Input: part model. Units: mm. Frame: model coordinates. A direction names the side the tool comes from. Round coordinates to 2 decimals unless told otherwise and drop trailing zeros. Order: outer loops, then holes, each group sorted by start corner. A loop starts at its lowest first (then second) coordinate and runs counter-clockwise, first axis right, second up. Notation, with made-up numbers: (70, 79) -> (113, 79) arc R33 ccw to (113, 108) -> close; hole circle Ø2 at (-18.5, -32). An arc over 180 degrees is marked (long way). Use a Markdown table: item, result.
from build123d import *

# Parameters (mm, degrees)
SKETCH_1_R            = 21.5
SKETCH_1_R_2          = 1.5
SKETCH_1_R_3          = 10
EXTRUDE_1_DEPTH       = 9
SHELL_4_T             = -2
EXTRUDE_2_OUTLINE_R   = 21.5
EXTRUDE_2_OUTLINE_R_2 = 1.5
EXTRUDE_2_OUTLINE_R_3 = 4
EXTRUDE_2_DEPTH       = 3
SKETCH_5_R            = 13.5
SKETCH_5_R_2          = 1.5
SKETCH_5_R_3          = 4
EXTRUDE_3_DEPTH       = 3


# Read off the part's stored shape, not the designer's step: 凸台-拉伸2
with BuildPart() as part:
    # 草图1 → 凸台-拉伸1 (new body)
    with BuildSketch(Plane(origin=(0, 0, 0), x_dir=(1, 0, 0), z_dir=(0, 1, 0))):
        with Locations(Location((0, 0, 0), (0, 0, 270))):
            Circle(SKETCH_1_R)
        with Locations(Location((12.374368671, 12.374368671, 0), (0, 0, 270))):
            Circle(SKETCH_1_R_2, mode=Mode.SUBTRACT)
        with Locations(Location((0, 0, 0), (0, 0, 270))):
            Circle(SKETCH_1_R_3, mode=Mode.SUBTRACT)
        with Locations(Location((12.374368671, -12.374368671, 0), (0, 0, 90))):
            Circle(SKETCH_1_R_2, mode=Mode.SUBTRACT)
        with Locations(Location((-12.374368671, -12.374368671, 0), (0, 0, 270))):
            Circle(SKETCH_1_R_2, mode=Mode.SUBTRACT)
        with Locations(Location((-12.374368671, 12.374368671, 0), (0, 0, 90))):
            Circle(SKETCH_1_R_2, mode=Mode.SUBTRACT)
        with Locations(Location((0, 17.5, 0), (0, 0, 90))):
            Circle(SKETCH_1_R_2, mode=Mode.SUBTRACT)
        with Locations(Location((17.5, 0, 0), (0, 0, 270))):
            Circle(SKETCH_1_R_2, mode=Mode.SUBTRACT)
        with Locations(Location((0, -17.5, 0), (0, 0, 90))):
            Circle(SKETCH_1_R_2, mode=Mode.SUBTRACT)
        with Locations(Location((-17.5, 0, 0), (0, 0, 270))):
            Circle(SKETCH_1_R_2, mode=Mode.SUBTRACT)
    extrude(amount=EXTRUDE_1_DEPTH)

    # 抽壳4
    shell_4_openings = [part.faces().sort_by_distance(p)[0] for p in [
        (0, 9, -20.891888168),
    ]]
    offset(amount=SHELL_4_T, openings=shell_4_openings, kind=Kind.INTERSECTION)

    # 凸台-拉伸2 outline → 凸台-拉伸2 (add)
    with BuildSketch(Plane(origin=(0, 9, 0), x_dir=(1, 0, 0), z_dir=(0, 1, 0))):
        Circle(EXTRUDE_2_OUTLINE_R)
        with Locations((-12.374368671, -12.374368671)):
            Circle(EXTRUDE_2_OUTLINE_R_2, mode=Mode.SUBTRACT)
        with Locations((0, -17.5)):
            Circle(EXTRUDE_2_OUTLINE_R_2, mode=Mode.SUBTRACT)
        with Locations((12.374368671, -12.374368671)):
            Circle(EXTRUDE_2_OUTLINE_R_2, mode=Mode.SUBTRACT)
        with Locations((0, -7)):
            Circle(EXTRUDE_2_OUTLINE_R_2, mode=Mode.SUBTRACT)
        with Locations((-17.5, 0)):
            Circle(EXTRUDE_2_OUTLINE_R_2, mode=Mode.SUBTRACT)
        with Locations((-7, 0)):
            Circle(EXTRUDE_2_OUTLINE_R_2, mode=Mode.SUBTRACT)
        with Locations((-12.374368671, 12.374368671)):
            Circle(EXTRUDE_2_OUTLINE_R_2, mode=Mode.SUBTRACT)
        Circle(EXTRUDE_2_OUTLINE_R_3, mode=Mode.SUBTRACT)
        with Locations((7, 0)):
            Circle(EXTRUDE_2_OUTLINE_R_2, mode=Mode.SUBTRACT)
        with Locations((0, 7)):
            Circle(EXTRUDE_2_OUTLINE_R_2, mode=Mode.SUBTRACT)
        with Locations((17.5, 0)):
            Circle(EXTRUDE_2_OUTLINE_R_2, mode=Mode.SUBTRACT)
        with Locations((0, 17.5)):
            Circle(EXTRUDE_2_OUTLINE_R_2, mode=Mode.SUBTRACT)
        with Locations((12.374368671, 12.374368671)):
            Circle(EXTRUDE_2_OUTLINE_R_2, mode=Mode.SUBTRACT)
    extrude(amount=EXTRUDE_2_DEPTH)

    # 草图5 → 凸台-拉伸3 (add)
    with BuildSketch(Plane(origin=(0, 12, 0), x_dir=(1, 0, 0), z_dir=(0, 1, 0))):
        with Locations(Location((0, 0, 0), (0, 0, 270))):
            Circle(SKETCH_5_R)
        with Locations(Location((-7, 0, 0), (0, 0, 270))):
            Circle(SKETCH_5_R_2, mode=Mode.SUBTRACT)
        with Locations(Location((0, -7, 0), (0, 0, 270))):
            Circle(SKETCH_5_R_2, mode=Mode.SUBTRACT)
        with Locations(Location((7, 0, 0), (0, 0, 270))):
            Circle(SKETCH_5_R_2, mode=Mode.SUBTRACT)
        with Locations(Location((0, 0, 0), (0, 0, 270))):
            Circle(SKETCH_5_R_3, mode=Mode.SUBTRACT)
        with Locations(Location((0, 7, 0), (0, 0, 270))):
            Circle(SKETCH_5_R_2, mode=Mode.SUBTRACT)
    extrude(amount=EXTRUDE_3_DEPTH)


solid = part.part
1) Set-up query: faces 5 (the face through (0.56, 12.62, 8.39)), 6 (the face through (18.04, 5.45, -7.4)), 7 (the face through (3, 15, 3)), 8 (the face through (-13.18, 13.48, -2.93)), 9 (the face through (-0.1, 9, 4.3)). Return all of +Z, -Z, +X, -X, +Y, -Y with unobstructed straight access to the full face (end or side cutting, diameter ignored); none if empty.
Answer key:
| item | result |
|---|---|
| face 5 | +Y, -Y |
| face 6 | none |
| face 7 | +Z, -Z, +X, -X, +Y |
| face 8 | +Y |
| face 9 | -Y |
2) Ray query, probe 1 along X at (y, z) = (13.65, 0); probe 2 along X at (y, z) = (10.35, 0); probe 3 along Y at (x, z) = (2, 13). Return the intervals inside material, ascending.
Answer key:
| item | result |
|---|---|
| probe 1 | x = -13.5 to -8.5, -5.5 to -4, 4 to 5.5, 8.5 to 13.5 |
| probe 2 | x = -21.5 to -19, -16 to -8.5, -5.5 to -4, 4 to 5.5, 8.5 to 16, 19 to 21.5 |
| probe 3 | y = 0 to 2, 9 to 15 |
3) Cut plane C-C on y = 10. State how many separate pieces and enclosed holes the cut face has, and give its area (3 significant figures).
Answer key:
| item | result |
|---|---|
| separate pieces | 1 |
| enclosed holes | 13 |
| area | 1,320 mm^2 |
4) Cut plane B-B on z = -17.5. Return loops of the section in (x, y), and give its area (3 significant figures).
Answer key:
| item | result |
|---|---|
| outline | (-12.49, 0) -> (-1.5, 0) -> (-1.5, 12) -> (-12.49, 12) -> close; (1.5, 0) -> (12.49, 0) -> (12.49, 12) -> (1.5, 12) -> close; hole (-8.6, 2) -> (-3.5, 2) -> (-3.5, 9) -> (-8.6, 9) -> close; hole (3.5, 2) -> (8.6, 2) -> (8.6, 9) -> (3.5, 9) -> close |
| area | 192 mm^2 |
5) Draft query along Y for faces 1 (the face through (-18.04, 5.45, 7.4)), 2 (the face through (-9.76, 4.44, -2.17)), 3 (the face through (-4.5, 0, 9.3)), 4 (the face through (18, 5.5, 7.5)). Return one class per face: released by +Y, released by -Y, zero draft, split by the parting line, or undercut.
Answer key:
| item | result |
|---|---|
| face 1 | undercut |
| face 2 | zero draft |
| face 3 | released by -Y |
| face 4 | undercut |
6) Cut plane A-A on x = -7. Return loops of the section in (y, z).
Answer key:
| item | result |
|---|---|
| outline | (0, -20.33) -> (12, -20.33) -> (12, -11.54) -> (15, -11.54) -> (15, -1.5) -> (9, -1.5) -> (9, -7.14) -> (0, -7.14) -> close; (0, 7.14) -> (9, 7.14) -> (9, 1.5) -> (15, 1.5) -> (15, 11.54) -> (12, 11.54) -> (12, 20.33) -> (0, 20.33) -> close; hole (2, -18.2) -> (9, -18.2) -> (9, -9.75) -> (2, -9.75) -> close; hole (2, 9.75) -> (9, 9.75) -> (9, 18.2) -> (2, 18.2) -> close |
7) Contact query for flat-ended pins moving along their axis: P1, Ø16, axis at x = 3, z = 1.5, coming from the -Y side; P2, Ø3, axis at x = 6, y = 11, coming from the +Z side; P3, Ø4, axis at x = -5, z = -16, coming from the +Y side; P4, Ø1, axis at x = -16.5, y = 3.5, coming from the +Z side. Output: stop coordinate, or through.
Answer key:
| item | result |
|---|---|
| P1 | stops at y = 0 |
| P2 | stops at z = 21.02 |
| P3 | stops at y = 12 |
| P4 | stops at z = 14.36 |
